from build123d import *

# Parameters (mm, degrees)
BOSS_EXTRU_1_DEPTH      = 40
EPAISSIR2_DEPTH         = 40
EPAISSIR3_DEPTH         = 40
ESQUISSE11_R            = 5
ENL_V_MAT_EXTRU_1_DEPTH = 10
ECHELLE1_SCALE          = 0.25


# Read off the part's stored shape, not the designer's step: Epaissir2, Epaissir3
with BuildPart() as part:
    # Esquisse1 → Boss.-Extru.1 (new body)
    with BuildSketch(Plane.XY):
        with BuildLine():
            Line((-85, 105), (-63.639838362, 126.360161638))
            Line((-63.639838362, 126.360161638), (63.639838362, 126.360161638))
            Line((63.639838362, 126.360161638), (85, 105))
            Line((85, 105), (85, -35))
            ThreePointArc((85, -35), (86.201897264, -45), (85, -55))
            Line((85, -55), (85, -65))
            ThreePointArc((85, -65), (83.535533906, -68.535533906), (80, -70))
            Line((80, -70), (-80, -70))
            ThreePointArc((-80, -70), (-83.535533906, -68.535533906), (-85, -65))
            Line((-85, -65), (-85, -55))
            ThreePointArc((-85, -55), (-86.201897264, -45), (-85, -35))
            Line((-85, -35), (-85, 105))
        make_face()
        with BuildLine():
            Line((75, 100.857864376), (59.497702738, 116.360161638))
            Line((59.497702738, 116.360161638), (-59.497702738, 116.360161638))
            Line((-59.497702738, 116.360161638), (-75, 100.857864376))
            Line((-75, 100.857864376), (-75, -36.284378696))
            ThreePointArc((-75, -36.284378696), (-76.201897264, -45), (-75, -53.715621304))
            Line((-75, -53.715621304), (-75, -60))
            Line((-75, -60), (75, -60))
            Line((75, -60), (75, -53.715621304))
            ThreePointArc((75, -53.715621304), (76.201897264, -45), (75, -36.284378696))
            Line((75, -36.284378696), (75, 100.857864376))
        make_face(mode=Mode.SUBTRACT)
    extrude(amount=BOSS_EXTRU_1_DEPTH)

    # Epaissir2 outline → Epaissir2 (add)
    with BuildSketch(Plane.XY):
        with BuildLine():
            ThreePointArc((-63.639838362, 126.360161638), (-77.097387468, 118.457549106), (-85, 105))
            Line((-85, 105), (-63.639838362, 126.360161638))
        make_face()
    extrude(amount=EPAISSIR2_DEPTH)

    # Epaissir3 outline → Epaissir3 (add)
    with BuildSketch(Plane.XY):
        with BuildLine():
            ThreePointArc((85, 105), (77.097387468, 118.457549106), (63.639838362, 126.360161638))
            Line((63.639838362, 126.360161638), (85, 105))
        make_face()
    extrude(amount=EPAISSIR3_DEPTH)

    # Esquisse11 → Enlèv. mat.-Extru.1 (cut)
    with BuildSketch(Plane(origin=(0, 126.360161638, 0), x_dir=(1, 0, 0), z_dir=(0, 1, 0))):
        with Locations(Location((0, -20, 0), (0, 0, 270))):
            Circle(ESQUISSE11_R)
    extrude(amount=-ENL_V_MAT_EXTRU_1_DEPTH, mode=Mode.SUBTRACT)


with BuildPart() as part_1:
    # Echelle1: scaled about (0, 26.941606469, 20)
    add(part.part.scale(ECHELLE1_SCALE).moved(Location((0, 20.206204852, 15))))


solid = part_1.part
Work out the finished part from the listing and answer in its coordinate system (mm). A direction names the side the tool comes from. Give positions to 0.01 mm unless a question says otherwise; leave off trailing zeros. Loops run counter-clockwise (first coordinate to the right, second up) from the corner with the lowest first, then second, coordinate; pieces in that order, holes last. Notation, with made-up numbers: (32.5, -17) -> (70.5, -17) arc R11 ccw to (70.5, -5) -> close; hole circle Ø1 at (-38.75, 80). An arc over 180 degrees is marked (long way). Use a Markdown table: item, result. Add a question column.
1) The part is cut by section B-B, the plane x = 0. Determine the outline of the cut face in (y, z).
2) Which of the six approach directions +Z, -Z, +X, -X, +Y, -Y give full straight-line access (tool end or side, diameter ignored) to faces 1 (the flat face through (-18.75, 6, 20)), 2 (the flat face through (21.25, 29, 20)), 3 (the cylindrical face through (-0.479, 50.564, 21.155)), 4 (the flat face through (-21.25, 5, 20))?
3) The part is cut by section D-D, the plane x = 17.5. Determine the outline of the cut face in (y, z).
4) For a pull along Y with two mould halves and no side action, classify faces 5 (the cylindrical face through (-21.55, 8.92, 19.93)), 6 (the flat face through (-21.25, 29, 20)), 7 (the flat face through (0, 51.796, 18)), 8 (the flat face through (0, 5.206, 20)) as +Y half, -Y half, draft (parallel to the pull), parting line (faces both ways), or undercut.
5) Each of these flat-tipped pins is pushed along its axis until it touches: P1, Ø1.2, axis at y = 5, z = 19.5, coming from the -X side; P2, Ø2, axis at y = 44, z = 21.5, coming from the +X side; P3, Ø3, axis at y = 5, z = 21, coming from the +X side. Where does it stop, or does it pass through?
6) The part is cut by section A-A, the plane y = 24.5. Determine the outline of the cut face in (x, z), plus the area to 3 significant figures.
7) The part is cut by section C-C, the plane z = 23.75. Determine the outline of the cut face in (x, y), plus the area to 3 significant figures.
8) Consider line 1 along Y through (x, z) = (7.5, 17); line 2 along X through (y, z) = (30, 16.25); line 3 along X through (y, z) = (51, 20). Determine where each line is inside the solid, lowest interval first.
Reported:
| question | item | result |
|---|---|---|
| 1 | outline | (2.71, 15) -> (5.21, 15) -> (5.21, 25) -> (2.71, 25) -> close; (49.3, 15) -> (51.8, 15) -> (51.8, 18.75) -> (49.3, 18.75) -> close; (49.3, 21.25) -> (51.8, 21.25) -> (51.8, 25) -> (49.3, 25) -> close |
| 2 | face 1 | +Z, -Z |
| 2 | face 2 | +Z, -Z, +X, +Y |
| 2 | face 3 | +Y |
| 2 | face 4 | +Z, -Z, -X, -Y |
| 3 | outline | (2.71, 15) -> (5.21, 15) -> (5.21, 25) -> (2.71, 25) -> close; (46.67, 15) -> (51.15, 15) -> (51.15, 25) -> (46.67, 25) -> close |
| 4 | face 5 | parting line |
| 4 | face 6 | draft |
| 4 | face 7 | +Y half |
| 4 | face 8 | undercut |
| 5 | P1 | stops at x = -21.25 |
| 5 | P2 | stops at x = 21.25 |
| 5 | P3 | stops at x = 21.26 |
| 6 | outline | (-21.25, 15) -> (-18.75, 15) -> (-18.75, 25) -> (-21.25, 25) -> close; (18.75, 15) -> (21.25, 15) -> (21.25, 25) -> (18.75, 25) -> close |
| 6 | area | 50.0 mm^2 |
| 7 | outline | (-21.25, 3.96) arc R1.25 ccw to (-20, 2.71) -> (20, 2.71) arc R1.25 ccw to (21.25, 3.96) -> (21.25, 6.46) arc R10.55 ccw to (21.25, 11.46) -> (21.25, 46.46) arc R7.75 ccw to (15.91, 51.8) -> (-15.91, 51.8) arc R7.75 ccw to (-21.25, 46.46) -> (-21.25, 11.46) arc R10.55 ccw to (-21.25, 6.46) -> close; hole (-18.75, 5.21) -> (18.75, 5.21) -> (18.75, 6.78) arc R8.05 ccw to (18.75, 11.14) -> (18.75, 45.42) -> (14.87, 49.3) -> (-14.87, 49.3) -> (-18.75, 45.42) -> (-18.75, 11.14) arc R8.05 ccw to (-18.75, 6.78) -> close |
| 7 | area | 429 mm^2 |
| 8 | line 1 | y = 2.71 to 5.21, 49.3 to 51.8 |
| 8 | line 2 | x = -21.25 to -18.75, 18.75 to 21.25 |
| 8 | line 3 | x = -17.76 to -1.25, 1.25 to 17.76 |
